from build123d import *

# Parameters (mm, degrees)
F1_DEPTH    = 5
F2_SIZE     = 3
F3_T1_DEPTH = 12.3553390593
F3_T3_DEPTH = 13.1207993933


# Not quite as in the source:
# - a fillet or chamfer that OpenCascade refuses, or shapes differently, is made with other operations: its cross-section is extruded or revolved along the edge and cut away or added


with BuildPart() as f1:
    # F0 (on Right) → F1 (new body, symmetric)
    with BuildSketch(Plane.YZ):
        with BuildLine():
            Line((11.971969828, -2), (11.971969828, 0))
            Line((11.971969828, 0), (-18.028030172, 0))
            ThreePointArc((-18.028030172, 0), (-20.0255447559, 2.0996769133), (-17.828924084, 3.990064513))
            Line((-17.828924084, 3.990064513), (2.0717210456, 1.9990036332))
            Line((2.0717210456, 1.9990036332), (2.1335235149, 2.6167190544))
            Line((2.1335235149, 2.6167190544), (-4.3118495071, 4.6476653855))
            Line((-4.3118495071, 4.6476653855), (-17.629817996, 5.9801290259))
            ThreePointArc((-17.629817996, 5.9801290259), (-22.0230593398, 2.1993538266), (-18.028030172, -2))
            Line((-18.028030172, -2), (11.971969828, -2))
        make_face()
    extrude(amount=F1_DEPTH, both=True)

    # F2
    f2_edges = [f1.edges().sort_by_distance(p)[0] for p in [
        (5, 11.97197, -1),
        (-5, 11.97197, -1),
    ]]
    chamfer(f2_edges, length=F2_SIZE)

    # F3: fillet of radius 5 on 6 edges, made by hand

    # F3_s2 → F3_t1 (cut)
    with BuildSketch(Plane.XY.offset(-7.1776695297)):
        with BuildLine():
            ThreePointArc((-3.5355339059, 10.4364359221), (-4.6193976626, 8.814319178), (-5, 6.9009020161))
            Line((-5, 6.9009020161), (-5, 8.971969828))
            Line((-5, 8.971969828), (-3.5355339059, 10.4364359221))
        make_face()
        with BuildLine():
            ThreePointArc((0.0710678119, 11.971969828), (-1.84234935, 11.5913674906), (-3.4644660941, 10.5075037339))
            Line((-3.4644660941, 10.5075037339), (-2, 11.971969828))
            Line((-2, 11.971969828), (0.0710678119, 11.971969828))
        make_face()
        with BuildLine():
            ThreePointArc((-0.0710678119, 11.971969828), (1.84234935, 11.5913674906), (3.4644660941, 10.5075037339))
            Line((3.4644660941, 10.5075037339), (2, 11.971969828))
            Line((2, 11.971969828), (-0.0710678119, 11.971969828))
        make_face()
        with BuildLine():
            ThreePointArc((3.5355339059, 10.4364359221), (4.6193976626, 8.814319178), (5, 6.9009020161))
            Line((5, 6.9009020161), (5, 8.971969828))
            Line((5, 8.971969828), (3.5355339059, 10.4364359221))
        make_face()
    extrude(amount=F3_T1_DEPTH, mode=Mode.SUBTRACT)

    # F3_s4 → F3_t3 (cut)
    with BuildSketch(Plane(origin=(0, 0.2185507121, 2.1844134494), x_dir=(1, 0, 0), z_dir=(0, 0.099553044, 0.9950322565))):
        with BuildLine():
            ThreePointArc((-5, -3.1375776299), (-3.5355339059, 0.3979562761), (0, 1.8624223701))
            Line((0, 1.8624223701), (-5, 1.8624223701))
            Line((-5, 1.8624223701), (-5, -3.1375776299))
        make_face()
        with BuildLine():
            ThreePointArc((5, -3.1375776299), (3.5355339059, 0.3979562761), (0, 1.8624223701))
            Line((0, 1.8624223701), (5, 1.8624223701))
            Line((5, 1.8624223701), (5, -3.1375776299))
        make_face()
    extrude(amount=F3_T3_DEPTH, mode=Mode.SUBTRACT)


solid = f1.part
The listing builds one solid part. Answer for the finished solid, in the listing's coordinates (mm). A direction names the side the tool comes from. Give positions to 0.01 mm unless a question says otherwise; leave off trailing zeros. Order: outer loops, then holes, each group sorted by start corner. A loop starts at its lowest first (then second) coordinate and runs counter-clockwise, first axis right, second up. Notation, with made-up numbers: (17.5, -27) - (56.5, -27) arc R23 cw to (56.5, -2) - close; hole circle Ø2 at (17.25, 64). An arc over 180 degrees is marked (long way). One line per item, written item: value. Start each with the question number.
1) The mould has two halves that part along Z. Classify faces 3 (the face through (0.07, -8.02, 3.01)), 4 (the face through (0.07, -20.027, 2.054)), 5 (the face through (1.85, 11.59, -1.01)), 6 (the face through (0.07, -22.018, 2.29)): released by +Z, released by -Z, zero draft, split by the parting line, or undercut.
2) A cutting plane is placed at A-A on y = -14. Give the vertices of the cut face in (x, z).
3) Find the intervals of material crossed by L1, parallel to Z at x = 3.5, y = -18; L2, parallel to Z at x = 0.5, y = 3.5; L3, parallel to Z at x = -0.75, y = -14, in increasing order.
4) A cutting plane is placed at C-C on z = -1. Give the vertices of the cut face in (x, y), then the cut area to 3 significant figures.
5) A cutting plane is placed at D-D on z = 1.5. Give the vertices of the cut face in (x, y).
6) A tool of negligible diameter and unlimited length cuts with its end or side. For faces 1 (the face through (0, -3, 0)), 2 (the face through (0.07, -1.76, 3.844)), from which of +Z, -Z, +X, -X, +Y, -Y can it reach the whole face along a straight path? Write none if from no direction.
7) A cutting plane is placed at B-B on x = -2.25. Give the vertices of the cut face in (y, z), then the cut area to 3 significant figures.
8) Given pin 1 Ø1 at (x, y) = (-0.5, -15.5) entering from +Z, flat-ended and moving along its own axis, determine where the tip first touches the part or whether it passes through.
Answer sheet:
1. face 3: undercut
1. face 4: undercut
1. face 5: zero draft
1. face 6: split by the parting line
2. outline: (-5, -2) - (5, -2) - (5, 0) - (-5, 0) - close; (-5, 3.61) - (5, 3.61) - (5, 5.62) - (-5, 5.62) - close
3. L1: z = -2 to 0, 4 to 6
3. L2: z = -2 to 0
3. L3: z = -2 to 0, 3.61 to 5.62
4. outline: (-5, -20.67) - (5, -20.67) - (5, 6.9) arc R5 ccw to (3.54, 10.44) - (3.46, 10.51) arc R5 ccw to (0, 11.97) arc R5 ccw to (-3.46, 10.51) - (-3.54, 10.44) arc R5 ccw to (-5, 6.9) - close
4. area: 315 mm2
5. outline: (-5, -22) - (5, -22) - (5, -19.96) - (-5, -19.96) - close
6. face 1: +X, -X, +Y
6. face 2: +Z, +X, -X, +Y
7. outline: (-18.03, -2) - (11.4, -2) - (11.4, 0) - (-18.03, 0) arc R2 cw (long way) to (-17.83, 3.99) - (1.54, 2.05) - (1.61, 2.78) - (-4.31, 4.65) - (-17.63, 5.98) arc R4 ccw (long way) to start
7. area: 113 mm2
8. pin 1: stops at z = 5.82
